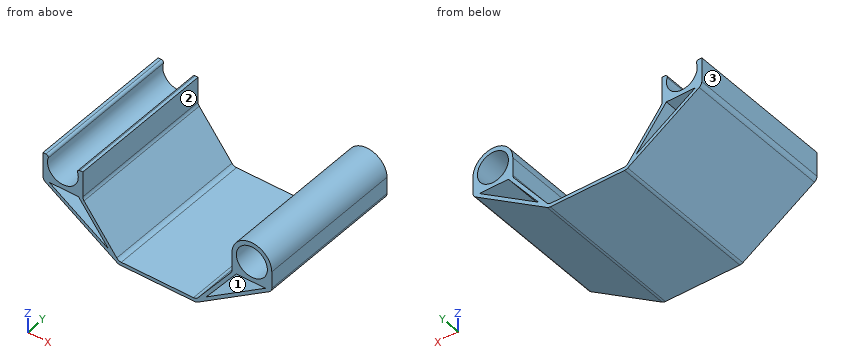
```python
from build123d import *

# Parameters (mm, degrees)
BOSS_EXTRUDE1_DEPTH = 130.5
SKETCH4_W           = 34.8
SKETCH4_H           = 34.8
SKETCH4_R           = 13.45
BOSS_EXTRUDE2_DEPTH = 130.5
FILLET1_R           = 5
CUT_EXTRUDE4_DEPTH  = 182.887575167
SKETCH6_R           = 13.55
CUT_EXTRUDE5_DEPTH  = 182.887575167


with BuildPart() as part:
    # Sketch1 → Boss-Extrude1 (new body)
    with BuildSketch(Plane(origin=(0, 0, 0), x_dir=(1, 0, 0), z_dir=(0, 1, 0))):
        with BuildLine():
            Line((0, 0), (-34, 0))
            Line((-34, 0), (-100, -43))
            Line((-100, -43), (-100, -66.97))
            Line((-100, -66.97), (-97.358644924, -66.97))
            ThreePointArc((-97.358644924, -66.97), (-95.748804634, -66.156766295), (-95.448140727, -64.378414239))
            ThreePointArc((-95.448140727, -64.378414239), (-82.6, -46.95), (-69.751859273, -64.378414239))
            ThreePointArc((-69.751859273, -64.378414239), (-69.451195366, -66.156766295), (-67.841355076, -66.97))
            Line((-67.841355076, -66.97), (-65.2, -66.97))
            Line((-65.2, -66.97), (-65.2, -43))
            Line((-65.2, -43), (-34, -3))
            Line((-34, -3), (0, -3))
            Line((0, -3), (0, 0))
        make_face()
        Polygon((-69.004681327, -43), (-94.504291462, -43), (-42.656655328, -9.220479488), align=None, mode=Mode.SUBTRACT)
    boss_extrude1 = extrude(amount=BOSS_EXTRUDE1_DEPTH)

    # Mirror1: Boss-Extrude1 across plane
    add(boss_extrude1.mirror(Plane(origin=(0, 130.5, 3), x_dir=(0, 0, 1), z_dir=(-1, 0, 0))))

    # Sketch4 → Boss-Extrude2 (add)
    with BuildSketch(Plane.XZ):
        with Locations((82.6, 60.4)):
            Rectangle(SKETCH4_W, SKETCH4_H)
        with Locations(Location((82.6, 60.4, 0), (0, 0, 270))):
            Circle(SKETCH4_R, mode=Mode.SUBTRACT)
    extrude(amount=-BOSS_EXTRUDE2_DEPTH)

    # Fillet1
    fillet1_edges = [part.edges().sort_by_distance(p)[0] for p in [
        (-34, 65.25, 3),
        (-65.2, 65.25, 43),
        (-100, 65.25, 43),
        (-34, 65.25, 0),
        (34, 65.25, 3),
        (65.2, 65.25, 43),
        (100, 65.25, 43),
        (34, 65.25, 0),
    ]]
    fillet(fillet1_edges, radius=FILLET1_R)

    # Sketch5 → Cut-Extrude4 (cut, through all)
    with BuildSketch(Plane.XZ):
        with BuildLine():
            Line((65.2, 60.4), (65.2, 77.8))
            Line((65.2, 77.8), (83.070170915, 82.404410021))
            Line((83.070170915, 82.404410021), (100, 77.8))
            Line((100, 77.8), (100, 60.4))
            ThreePointArc((100, 60.4), (82.6, 77.8), (65.2, 60.4))
        make_face()
    extrude(amount=-CUT_EXTRUDE4_DEPTH, mode=Mode.SUBTRACT)

    # Sketch6 → Cut-Extrude5 (cut, through all)
    with BuildSketch(Plane.XZ):
        with Locations(Location((82.6, 60.4, 0), (0, 0, 270))):
            Circle(SKETCH6_R)
    extrude(amount=-CUT_EXTRUDE5_DEPTH, mode=Mode.SUBTRACT)


solid = part.part
```
Here's how the part is built. I have some questions about the finished solid (model axes, mm). Face numbers are marked on the shaded views. A direction names the side the tool comes from. Round coordinates to 2 decimals unless told otherwise and drop trailing zeros. Write each loop counter-clockwise with the first axis right and the second up, starting at its lowest first coordinate (ties: lowest second). Pieces come first, ordered by that corner, then holes.
Q1. If we section it at C-C on z = 37: Write out the boundary of the cut face in (x, y), plus the area to 3 significant figures.
Q2. Will these pins go through, and if not, where does the flat tip stop? P1, Ø1, axis at y = 38.5, z = 40, coming from the +X side; P2, Ø12, axis at y = 23, z = 19, coming from the -X side; P3, Ø12.5, axis at x = 85.5, y = 87, coming from the -Z side.
Q3. Which directions (+Z, -Z, +X, -X, +Y, -Y) give clear straight access to the entire face, cutting with the end or side of a thin tool? Please do the marked faces 1, 2 and 3.
Q4. If we section it at D-D on x = -82.6: Write out the boundary of the cut face in (y, z).
Q5. If we section it at B-B on x = 82.6: Write out the boundary of the cut face in (y, z), plus the area to 3 significant figures.
Q6. Please list where these lines run through material, in increasing order: probe 1 along X at (y, z) = (80.5, 60.4); probe 2 along X at (y, z) = (117.5, 26.5); probe 3 along Z at (x, y) = (74.5, 72.5).
Q7. If we section it at A-A on y = 26.5: Give the number of separate pieces and of enclosed holes in the cut face, plus the area to 3 significant figures.
Answer below:
1. outline: (-90.79, 0) - (-85.29, 0) - (-85.29, 130.5) - (-90.79, 130.5) - close; (-64.32, 0) - (-60.52, 0) - (-60.52, 130.5) - (-64.32, 130.5) - close; (60.52, 0) - (64.32, 0) - (64.32, 130.5) - (60.52, 130.5) - close; (85.29, 0) - (90.79, 0) - (90.79, 130.5) - (85.29, 130.5) - close
1. area: 2,430 mm2
2. P1: stops at x = 96.16
2. P2: stops at x = -72.37
2. P3: stops at z = 29.48
3. face 1: +Y, -Y
3. face 2: +Z, +Y, -Y
3. face 3: +Z, -Z, -X, +Y, -Y
4. outline: (0, 31.66) - (130.5, 31.66) - (130.5, 35.24) - (0, 35.24) - close; (0, 43) - (130.5, 43) - (130.5, 46.95) - (0, 46.95) - close
5. outline: (0, 31.66) - (130.5, 31.66) - (130.5, 35.24) - (0, 35.24) - close; (0, 43) - (130.5, 43) - (130.5, 46.85) - (0, 46.85) - close; (0, 73.95) - (130.5, 73.95) - (130.5, 77.8) - (0, 77.8) - close
5. area: 1,470 mm2
6. probe 1: x = -100 to -96.05, -69.15 to -65.2, 65.2 to 69.05, 96.15 to 100
6. probe 2: x = -74.67 to -69.18, -56.13 to -52.33, 52.33 to 56.13, 69.18 to 74.67
6. probe 3: z = 26.39 to 29.97, 43 to 49.54, 71.26 to 75.8
7. separate pieces: 1
7. enclosed holes: 3
7. area: 1,810 mm2
